from build123d import *

# Parameters (mm, degrees)
F0_W     = 101
F0_H     = 80
F1_DEPTH = 70
F3_DEPTH = 69
F5_DEPTH = 2
F7_DEPTH = 14
F8_R     = 5
F9_R     = 0.49999


# Not quite as in the source:
# - a fillet or chamfer is up to 0.001 mm smaller than in the source, because OpenCascade refuses the exact size


with BuildPart() as f1:
    # F0 (on Top) → F1 (new body)
    with BuildSketch(Plane.XY):
        Rectangle(F0_W, F0_H)
    extrude(amount=F1_DEPTH)

    # F2 (on face) → F3 (cut)
    with BuildSketch(Plane.XY.offset(70)):
        Polygon((48.5, 39), (-49.5, 39), (-49.5, 20.586034283), (-49.5, -39), (48.5, -39), (48.5, -30.7030728576), align=None)
    extrude(amount=-F3_DEPTH, mode=Mode.SUBTRACT)

    # F4 (on face) → F5 (cut)
    with BuildSketch(Plane.YZ.offset(50.5)):
        Polygon((38, 2), (38, 70), (-38, 70), (-38, 42.2970801592), (-38, 2), align=None)
    extrude(amount=-F5_DEPTH, mode=Mode.SUBTRACT)

    # F6 (on face) → F7 (join)
    with BuildSketch(Plane(origin=(48.5, 0, 0), x_dir=(0, -1, 0), z_dir=(-1, 0, 0))):
        Polygon((39, 1), (39, 70), (38, 70), (38, 2), (-38, 2), (-38, 70), (-39, 70), (-39, 1), align=None)
    extrude(amount=-F7_DEPTH)

    # F8
    f8_edges = [f1.edges().sort_by_distance(p)[0] for p in [
        (-0.5, 39, 1),
        (-49.5, 0, 1),
        (-0.5, -39, 1),
        (0, 40, 0),
        (-50.5, 0, 0),
        (0, -40, 0),
        (-50.5, -40, 35),
        (-50.5, 40, 35),
        (-49.5, 39, 35.5),
        (-49.5, -39, 35.5),
        (56.5, 39, 1),
        (56.5, -39, 1),
        (55.5, -38, 2),
        (55.5, 38, 2),
    ]]
    fillet(f8_edges, radius=F8_R)

    # F9 (radius 0.5 in the source; OpenCascade refuses exactly that, so slightly less here)
    f9_edges = [f1.edges().sort_by_distance(p)[0] for p in [
        (2.5, 40, 70),
        (-49.035534, 38.535534, 70),
        (50.5, 39.5, 70),
        (-50.5, 0, 70),
        (56.5, 39, 70),
        (-49.035534, -38.535534, 70),
        (62.5, 38.5, 70),
        (2.5, -40, 70),
        (55.5, 38, 70),
        (50.5, -39.5, 70),
        (48.5, 38.5, 70),
        (56.5, -39, 70),
        (2, 39, 70),
        (62.5, -38.5, 70),
        (-48.035534, 37.535534, 70),
        (55.5, -38, 70),
        (-49.5, 0, 70),
        (48.5, -38.5, 70),
        (-48.035534, -37.535534, 70),
        (2, -39, 70),
        (62.5, -39, 38),
        (62.5, -37.535534, 2.464466),
        (62.5, 0, 1),
        (62.5, -38, 38.5),
        (62.5, 37.535534, 2.464466),
        (62.5, -36.535534, 3.464466),
        (62.5, 39, 38),
        (62.5, 0, 2),
        (62.5, 36.535534, 3.464466),
        (62.5, 38, 38.5),
    ]]
    fillet(f9_edges, radius=F9_R)


solid = f1.part
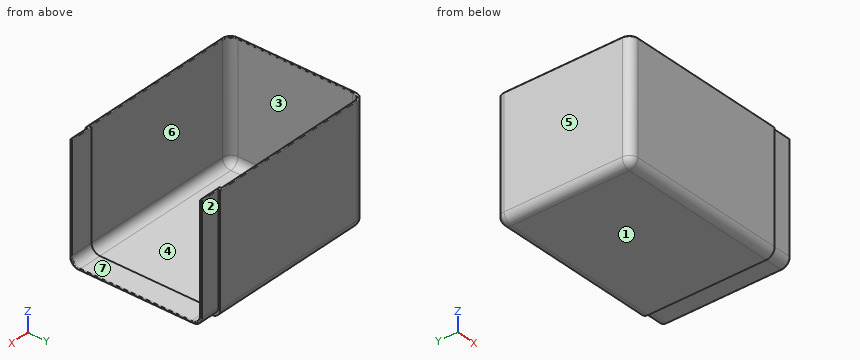
Read the model definition and answer for the solid it produces. Units are mm, in the model's axes. Face numbers are marked on the shaded views. A direction names the side the tool comes from. Round coordinates to 2 decimals unless told otherwise and drop trailing zeros.
1) The mould has two halves that part along X. Classify the marked faces 4, 5, 6 and 7: released by +X, released by -X, zero draft, split by the parting line, or undercut.
2) Straight lines are drawn through the part: L1, parallel to Y at x = -41, z = 8.5; L2, parallel to Z at x = 49.5, y = 29.5; L3, parallel to X at y = 9.5, z = 39. For each, find the intervals that lie inside material, in ascending order.
3) For the marked faces 1, 2 and 3, determine the directions among +Z, -Z, +X, -X, +Y, -Y from which every point of the face is accessible in a straight line to the end or side of a thin tool.
4) Flat-ended cylindrical pins translate along their axes: pin 1 (4 mm diameter, centred on x = 55, z = 28.5, fed in from -Y); pin 2 (8 mm diameter, centred on y = -31, z = 39, fed in from +X); pin 3 (8 mm diameter, centred on x = -16.5, y = -29.5, fed in from +Z). Find the tip coordinate at first contact, or state that the pin passes through.
Resolved:
1. face 4: undercut
1. face 5: released by -X
1. face 6: undercut
1. face 7: zero draft
2. L1: y = -40 to -39, 39 to 40
2. L2: z = 0 to 2
2. L3: x = -50.5 to -49.5
3. face 1: -Z, +X, -X, +Y, -Y
3. face 2: +Z, -Z, +X, +Y
3. face 3: +Z, +X
4. pin 1: stops at y = -39
4. pin 2: stops at x = -49.4
4. pin 3: stops at z = 1
